```python
from build123d import *

# Parameters (mm, degrees)
SKETCH1_R           = 22.8092
BOSS_EXTRUDE1_DEPTH = 23.8125
SKETCH2_OUTSIDE_W   = 102.245
SKETCH2_OUTSIDE_H   = 92.744
SKETCH2_OUTSIDE_R   = 30.707875178
CUT_EXTRUDE1_DEPTH  = 2.54
CUT_EXTRUDE1_TAPER  = 63


with BuildPart() as part:
    # Sketch1 → Boss-Extrude1 (new body)
    with BuildSketch(Plane.XY):
        Polygon((129.341403954, 1350.513952992), (147.070603954, 1319.806077815), (182.529003954, 1319.806077815), (200.258203954, 1350.513952992), (182.529003954, 1381.22182817), (147.070603954, 1381.22182817), align=None)
        with Locations((164.799803954, 1350.513952992)):
            Circle(SKETCH1_R, mode=Mode.SUBTRACT)
    extrude(amount=BOSS_EXTRUDE1_DEPTH)

    # Sketch2 outside → Cut-Extrude1 (cut)
    with BuildSketch(Plane.XY.offset(23.8125)):
        with Locations((164.7995, 1350.514)):
            Rectangle(SKETCH2_OUTSIDE_W, SKETCH2_OUTSIDE_H)
        with Locations((164.799803954, 1350.513952992)):
            Circle(SKETCH2_OUTSIDE_R, mode=Mode.SUBTRACT)
    extrude(amount=-CUT_EXTRUDE1_DEPTH, taper=CUT_EXTRUDE1_TAPER, mode=Mode.SUBTRACT)


solid = part.part
```
CAD build for the part. Positions are in the model's coordinates, mm. Coordinates: 2 decimals unless noted, no trailing zeros. Order: outer loops, then holes, each group sorted by start corner. A loop starts at its lowest first (then second) coordinate and runs counter-clockwise, first axis right, second up. Notation, with made-up numbers: (-18, -22.5) - (-12, -22.5) arc R24 cw to (-12, 3.5) - close; hole circle Ø4 at (19.5, -28.5). An arc over 180 degrees is marked (long way). Use a Markdown table: item, result. Add a question column.
(1) Saw through at A-A (z = 18.75). Give the cut face in (x, y), then the cut area to 3 significant figures.
(2) Pull direction X, two halves, no side cores. Call faces 1 (the face through (180.799, 1322.959, 23.224)), 2 (the face through (165, 1319.806, 12)), 3 (the face through (138.082, 1335.375, 11.74)), 4 (the face through (161.83, 1373.13, 11.74)): +X half, -X half, draft (parallel to the pull), parting line (faces both ways), or undercut.
(3) Flat gauge pins, fed straight in: pin 1 (3 mm diameter, centred on x = 189.5, z = 10.5, fed in from +Y); pin 2 (1 mm diameter, centred on x = 146.5, z = 18, fed in from +Y); pin 3 (2 mm diameter, centred on x = 143.5, z = 6.5, fed in from -Y). Where does each tip first touch, or does it go through?
(4) Drill centre lines: line 1 along X through (y, z) = (1349.5, 17.75); line 2 along Y through (x, z) = (177, 21.25); line 3 along X through (y, z) = (1346.5, 15.5). Where is each one in solid material? Low to high. Write a range as [from, to].
Solved:
| question | item | result |
|---|---|---|
| 1 | outline | (129.34, 1350.51) - (147.07, 1319.81) - (182.53, 1319.81) - (200.26, 1350.51) - (182.53, 1381.22) - (147.07, 1381.22) - close; hole circle Ø45.62 at (164.8, 1350.51) |
| 1 | area | 1,630 mm² |
| 2 | face 1 | +X half |
| 2 | face 2 | draft |
| 2 | face 3 | -X half |
| 2 | face 4 | undercut |
| 3 | pin 1 | stops at y = 1371.75 |
| 3 | pin 2 | stops at y = 1381.1 |
| 3 | pin 3 | stops at y = 1324.26 |
| 4 | line 1 | x = [129.93, 142.01], [187.59, 199.67] |
| 4 | line 2 | y = [1319.81, 1331.24], [1369.79, 1381.22] |
| 4 | line 3 | x = [131.66, 142.35], [187.25, 197.94] |
